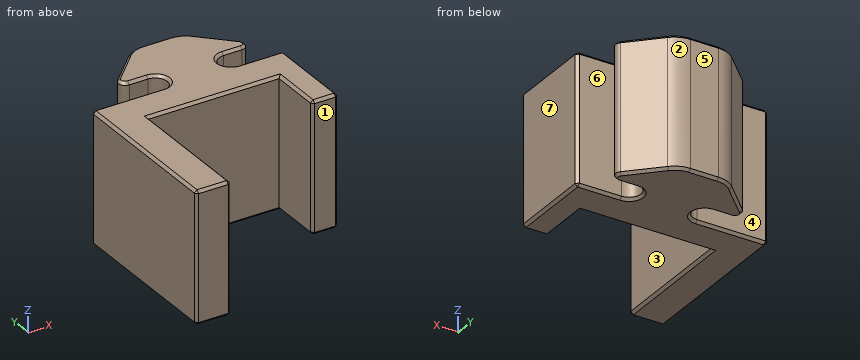
from build123d import *

# Parameters (mm, degrees)
BOSS_EXTRUDE1_DEPTH = 15
SKETCH2_W           = 4
SKETCH2_H           = 15
BOSS_EXTRUDE2_DEPTH = 15
SKETCH3_W           = 3
SKETCH3_H           = 15
BOSS_EXTRUDE3_DEPTH = 6
CHAMFER1_SIZE       = 0.3


with BuildPart() as part:
    # Sketch1 → Boss-Extrude1 (new body)
    with BuildSketch(Plane.XY):
        with BuildLine():
            Line((4.343399971, -3.3621), (5.0570836, -3.3621))
            Line((5.0570836, -3.3621), (9.5, -3.3621))
            Line((9.5, -3.3621), (9.5, -7.3621))
            Line((9.5, -7.3621), (-12.5, -7.3621))
            Line((-12.5, -7.3621), (-12.5, -3.3621))
            Line((-12.5, -3.3621), (-5.0570836, -3.3621))
            Line((-5.0570836, -3.3621), (-4.3434, -3.3621))
            ThreePointArc((-4.3434, -3.3621), (-2.9785, -1.9972), (-4.3434, -0.6323))
            Line((-4.3434, -0.6323), (-6.474794456, -0.6323))
            ThreePointArc((-6.474794456, -0.6323), (-7.173247382, -0.165608675), (-7.009367182, 0.658272727))
            Line((-7.009367182, 0.658272727), (-3.679323642, 3.988316267))
            ThreePointArc((-3.679323642, 3.988316267), (-2.73362958, 4.620208837), (-1.618107374, 4.8421))
            Line((-1.618107374, 4.8421), (1.618107374, 4.8421))
            ThreePointArc((1.618107374, 4.8421), (2.73362958, 4.620208837), (3.679323642, 3.988316267))
            Line((3.679323642, 3.988316267), (7.009367182, 0.658272727))
            ThreePointArc((7.009367182, 0.658272727), (7.173247382, -0.165608675), (6.474794456, -0.6323))
            Line((6.474794456, -0.6323), (4.343399971, -0.6323))
            ThreePointArc((4.343399971, -0.6323), (2.978499971, -1.9972), (4.343399971, -3.3621))
        make_face()
    extrude(amount=BOSS_EXTRUDE1_DEPTH)

    # Sketch2 → Boss-Extrude2 (add)
    with BuildSketch(Plane.XZ.offset(7.3621)):
        with Locations((-10.5, 7.5)):
            Rectangle(SKETCH2_W, SKETCH2_H)
    extrude(amount=BOSS_EXTRUDE2_DEPTH)

    # Sketch3 → Boss-Extrude3 (add)
    with BuildSketch(Plane.XZ.offset(7.3621)):
        with Locations((8, 7.5)):
            Rectangle(SKETCH3_W, SKETCH3_H)
    extrude(amount=BOSS_EXTRUDE3_DEPTH)

    # Chamfer1
    chamfer1_edges = [part.edges().sort_by_distance(p)[0] for p in [
        (9.5, -8.3621, 15),
        (-8.4217, -3.3621, 0),
        (-2.9785, -1.9972, 0),
        (-5.409097228, -0.6323, 0),
        (-7.173247382, -0.165608675, 0),
        (-5.344345412, 2.323294497, 0),
        (-2.73362958, 4.620208837, 0),
        (0, 4.8421, 0),
        (2.73362958, 4.620208837, 0),
        (5.344345412, 2.323294497, 0),
        (6.921699986, -3.3621, 15),
        (7.173247382, -0.165608675, 0),
        (5.409097213, -0.6323, 0),
        (2.978499971, -1.9972, 0),
        (6.921699986, -3.3621, 0),
        (9.5, -8.3621, 0),
        (-12.5, -12.8621, 0),
        (2.978499971, -1.9972, 15),
        (9.5, -3.3621, 7.5),
        (-12.5, -3.3621, 7.5),
        (5.409097213, -0.6323, 15),
        (7.173247382, -0.165608675, 15),
        (5.344345412, 2.323294497, 15),
        (2.73362958, 4.620208837, 15),
        (0, 4.8421, 15),
        (-8.4217, -3.3621, 15),
        (-1, -7.3621, 0),
        (-1, -7.3621, 15),
        (-2.73362958, 4.620208837, 15),
        (-8.5, -14.8621, 0),
        (-8.5, -14.8621, 15),
        (-12.5, -22.3621, 7.5),
        (-10.5, -22.3621, 0),
        (-8.5, -22.3621, 7.5),
        (-10.5, -22.3621, 15),
        (-5.344345412, 2.323294497, 15),
        (-7.173247382, -0.165608675, 15),
        (-5.409097228, -0.6323, 15),
        (6.5, -10.3621, 15),
        (6.5, -10.3621, 0),
        (9.5, -13.3621, 7.5),
        (8, -13.3621, 15),
        (6.5, -13.3621, 7.5),
        (8, -13.3621, 0),
        (-2.9785, -1.9972, 15),
        (-12.5, -12.8621, 15),
    ]]
    chamfer(chamfer1_edges, length=CHAMFER1_SIZE)


solid = part.part
Design review of the part built by this model. Coordinates are the model's own, in mm. Face numbers are marked on the shaded views. A direction names the side the tool comes from. Give positions to 0.01 mm unless a question says otherwise; leave off trailing zeros. Loops run counter-clockwise (first coordinate to the right, second up) from the corner with the lowest first, then second, coordinate; pieces in that order, holes last. Notation, with made-up numbers: (0, 85.25) - (11, 85.25) arc R22 ccw to (11, 105.25) - close; hole circle Ø5 at (26.5, -39). An arc over 180 degrees is marked (long way). Write item = value, one per line.
1) Take a section at D-D on x = 0.75. State the section outline as (y, z) points.
Result sheet:
outline = (-7.36, 0.3) - (-7.06, 0) - (4.54, 0) - (4.84, 0.3) - (4.84, 14.7) - (4.54, 15) - (-7.06, 15) - (-7.36, 14.7) - close
2) To check wall thickness, follow line 1 (X direction, y = -11.5, z = 3); line 2 (Y direction, x = 1.25, z = 2.5); line 3 (Y direction, x = -5.5, z = 5). State the ranges of each line that lie inside material, in increasing order.
Result sheet:
line_1 = -12.5 to -8.5, 6.5 to 9.5
line_2 = -7.36 to 4.84
line_3 = -7.36 to -3.36, -0.63 to 2.17
3) Tool access review of the marked faces 1, 2 and 3: name each direction out of +Z, -Z, +X, -X, +Y, -Y from which nothing blocks a thin tool from reaching the whole face with its end or side.
Result sheet:
face_1 = +Z, -Z, +X, -Y
face_2 = +Z, -Z, +X, +Y
face_3 = +Z, -Z, -Y
4) Take a section at A-A on y = -11.75. State the section outline as (x, z) points, and give its area (3 significant figures).
Result sheet:
outline = (-12.5, 0.3) - (-12.2, 0) - (-8.8, 0) - (-8.5, 0.3) - (-8.5, 14.7) - (-8.8, 15) - (-12.2, 15) - (-12.5, 14.7) - close; (6.5, 0.3) - (6.8, 0) - (9.2, 0) - (9.5, 0.3) - (9.5, 14.7) - (9.2, 15) - (6.8, 15) - (6.5, 14.7) - close
area = 105 mm2
5) Take a section at B-B on x = -5.5. State the section outline as (y, z) points.
Result sheet:
outline = (-7.36, 0.3) - (-7.06, 0) - (-3.66, 0) - (-3.36, 0.3) - (-3.36, 14.7) - (-3.66, 15) - (-7.06, 15) - (-7.36, 14.7) - close; (-0.63, 0.3) - (-0.33, 0) - (1.74, 0) - (2.17, 0.3) - (2.17, 14.7) - (1.74, 15) - (-0.33, 15) - (-0.63, 14.7) - close
6) Draft analysis for pull direction Y (two halves, no side actions). For the marked faces 4, 5, 6 and 7, state which applies: +Y half, -Y half, draft (parallel to the pull), parting line (faces both ways), or undercut.
Result sheet:
face_4 = undercut
face_5 = +Y half
face_6 = undercut
face_7 = draft
7) Take a section at C-C on z = 3.5. State the section outline as (x, y) points (3 decimals), and give its area (3 significant figures).
Result sheet:
outline = (-12.5, -22.062) - (-12.2, -22.362) - (-8.8, -22.362) - (-8.5, -22.062) - (-8.5, -7.362) - (6.5, -7.362) - (6.5, -13.062) - (6.8, -13.362) - (9.2, -13.362) - (9.5, -13.062) - (9.5, -3.662) - (9.2, -3.362) - (4.343, -3.362) arc R1.365 cw to (4.343, -0.632) - (6.475, -0.632) arc R0.756 ccw to (7.009, 0.658) - (3.679, 3.988) arc R2.915 ccw to (1.618, 4.842) - (-1.618, 4.842) arc R2.915 ccw to (-3.679, 3.988) - (-7.009, 0.658) arc R0.756 ccw to (-6.475, -0.632) - (-4.343, -0.632) arc R1.365 cw to (-4.343, -3.362) - (-12.2, -3.362) - (-12.5, -3.662) - close
area = 243 mm2
8) Clearance check with flat-ended pins moving along their axes: pin 1 Ø6.5 at (x, z) = (-8.5, 9.5) entering from +Y; pin 2 Ø3 at (y, z) = (-2, 9) entering from -X; pin 3 Ø2 at (x, z) = (-10, 11) entering from +Y. State where each tip first meets the part, or that it passes through.
Result sheet:
pin_1 = 2.42
pin_2 = -12.34
pin_3 = -3.36
